Print and shaded views of the part. All mm, measured from the part's lowest x, y and z. A direction names the side the tool comes from. Round coordinates to 2 decimals unless told otherwise and drop trailing zeros. Order: outer loops, then holes, each group sorted by start corner. A loop starts at its lowest first (then second) coordinate and runs counter-clockwise, first axis right, second up. Notation, with made-up numbers: M 42,-27.75 L 73,-27.75 A16 cw 73,-11.75 Z; hole C 31,12 d8. An arc over 180 degrees is marked long. Write each question's results on one line, items separated by ' | '. Start each with the question number.
1. Which spindle directions (+Z, -Z, +X, -X, +Y, -Y) get a long thin tool onto all of the face, cutting with end or side? Do the marked faces 5 and 6. Say none if no direction does.
2. Two-plate mould, pull along X, no slides. Class the marked faces 1, 2, 3 and 4: +X half, -X half, draft (parallel to the pull), parting line (faces both ways), or undercut.
3. Band-saw the part on A-A, the plane x = 50.8. List the corners of the cut face in (y, z).
4. Drop flat-ended pins along their axis: pin 1 Ø1 at (x, y) = (49.5, 2.5) entering from -Z; pin 2 Ø3 at (y, z) = (2, 15) entering from +X. Give the stop position or say it passes through.
5. Band-saw the part on B-B, the plane z = 12. List the corners of the cut face in (x, y).
6. Band-saw the part on C-C, the plane y = 3.2. List the corners of the cut face in (x, z) (1 decimal), then the cut area to 3 significant figures.
7. Band-saw the part on D-D, the plane z = 50.8. List the corners of the cut face in (x, y).
8. Probe L1, parallel to Z at x = 12.7, y = 2.1; L2, parallel to X at y = 4.5, z = 50.5; L3, parallel to X at y = 2.95, z = 50.8. List the from-to ranges inside material, lowest first. Write a range as [from, to].
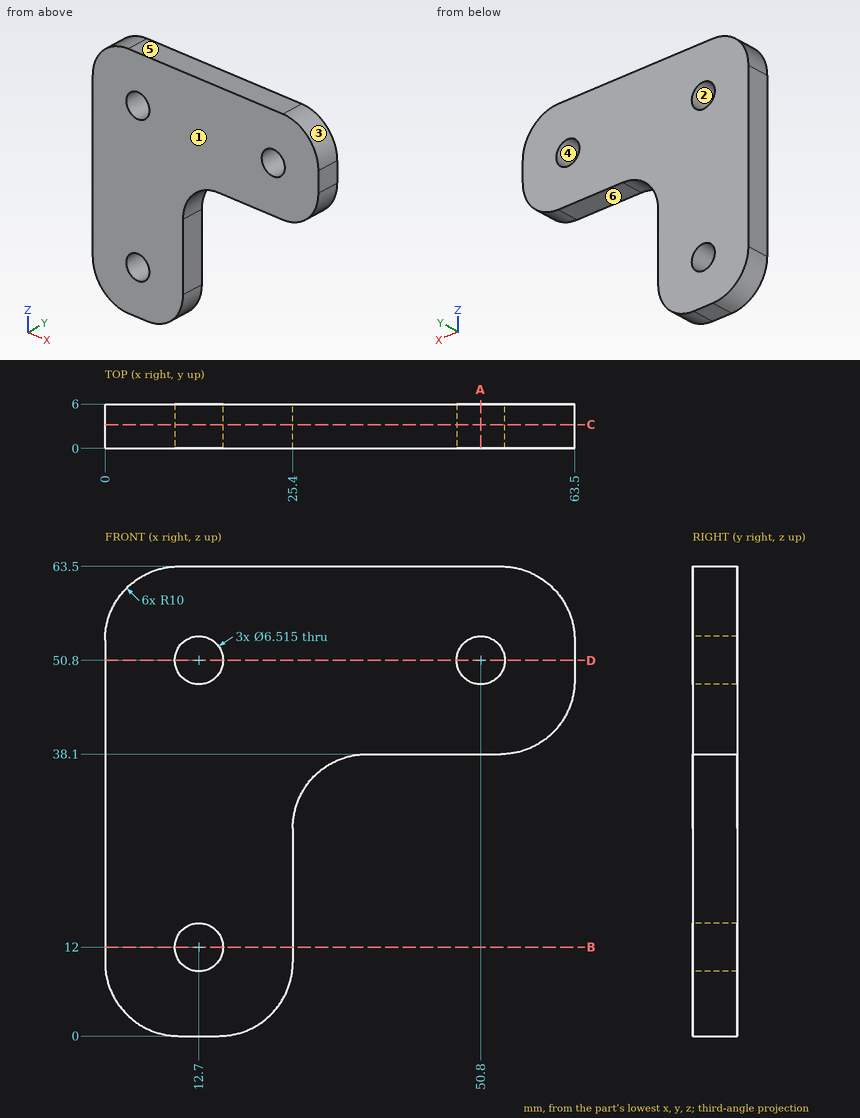
Solution:
1) face 5: +Z, +X, -X, +Y, -Y | face 6: -Z, +X, +Y, -Y
2) face 1: draft | face 2: undercut | face 3: +X half | face 4: undercut
3) outline: M 0,38.1 L 6,38.1 L 6,47.54 L 0,47.54 Z; M 0,54.06 L 6,54.06 L 6,63.5 L 0,63.5 Z
4) pin 1: z = 38.1 | pin 2: x = 25.4
5) outline: M 0,0 L 9.44,0 L 9.44,6 L 0,6 Z; M 15.96,0 L 25.4,0 L 25.4,6 L 15.96,6 Z
6) outline: M 0,10 A10 ccw 10,0 L 15.4,0 A10 ccw 25.4,10 L 25.4,28.1 A10 cw 35.4,38.1 L 53.5,38.1 A10 ccw 63.5,48.1 L 63.5,53.5 A10 ccw 53.5,63.5 L 10,63.5 A10 ccw 0,53.5 Z; hole C 12.7,12 d6.5; hole C 12.7,50.8 d6.5; hole C 50.8,50.8 d6.5 | area: 2,390 mm^2
7) outline: M 0,0 L 9.44,0 L 9.44,6 L 0,6 Z; M 15.96,0 L 47.54,0 L 47.54,6 L 15.96,6 Z; M 54.06,0 L 63.5,0 L 63.5,6 L 54.06,6 Z
8) L1: [0, 8.74], [15.26, 47.54], [54.06, 63.5] | L2: [0, 9.46], [15.94, 47.56], [54.04, 63.5] | L3: [0, 9.44], [15.96, 47.54], [54.06, 63.5]
